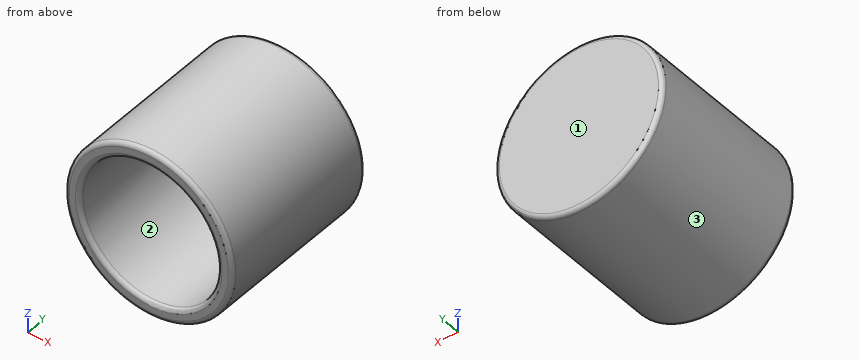
from build123d import *

# Parameters (mm, degrees)
F0_R     = 25.4
F0_R_2   = 20.955
F2_DEPTH = 50.8
F1_R     = 20.955
F3_DEPTH = 12.7
F4_R     = 1.27
F5_R     = 1.27
F6_R     = 1.27


with BuildPart() as f2:
    # F0 (on Front) → F2 (new body)
    with BuildSketch(Plane.XZ):
        Circle(F0_R)
        Circle(F0_R_2, mode=Mode.SUBTRACT)
    extrude(amount=F2_DEPTH)

    # F1 (on face) → F3 (join)
    with BuildSketch(Plane.XZ):
        Circle(F1_R)
    extrude(amount=F3_DEPTH)

    # F4
    f4_edges = [f2.edges().sort_by_distance(p)[0] for p in [
        (-25.4, -50.8, 0),
    ]]
    fillet(f4_edges, radius=F4_R)

    # F5
    f5_edges = [f2.edges().sort_by_distance(p)[0] for p in [
        (-20.955, -50.8, 0),
    ]]
    fillet(f5_edges, radius=F5_R)

    # F6
    f6_edges = [f2.edges().sort_by_distance(p)[0] for p in [
        (-25.4, 0, 0),
    ]]
    fillet(f6_edges, radius=F6_R)


solid = f2.part
Part model, mm, in its own coordinate system. Face numbers are marked on the shaded views. Give positions to 0.01 mm unless a question says otherwise; leave off trailing zeros. Loops run counter-clockwise (first coordinate to the right, second up) from the corner with the lowest first, then second, coordinate; pieces in that order, holes last.
(1) Band-saw the part on B-B (x = 0). Write the cut outline in (y, z) (3 decimals), and give its area (3 significant figures).
Return value:
outline: (-50.8, -24.13) arc R1.27 ccw to (-49.53, -25.4) - (-1.27, -25.4) arc R1.27 ccw to (0, -24.13) - (0, 24.13) arc R1.27 ccw to (-1.27, 25.4) - (-49.53, 25.4) arc R1.27 ccw to (-50.8, 24.13) - (-50.8, 22.225) arc R1.27 ccw to (-49.53, 20.955) - (-12.7, 20.955) - (-12.7, -20.955) - (-49.53, -20.955) arc R1.27 ccw to (-50.8, -22.225) - close
area: 982 mm2
(2) Band-saw the part on A-A (z = 0). Write the cut outline in (x, y) (3 decimals).
Return value:
outline: (-25.4, -49.53) arc R1.27 ccw to (-24.13, -50.8) - (-22.225, -50.8) arc R1.27 ccw to (-20.955, -49.53) - (-20.955, -12.7) - (20.955, -12.7) - (20.955, -49.53) arc R1.27 ccw to (22.225, -50.8) - (24.13, -50.8) arc R1.27 ccw to (25.4, -49.53) - (25.4, -1.27) arc R1.27 ccw to (24.13, 0) - (-24.13, 0) arc R1.27 ccw to (-25.4, -1.27) - close
(3) Band-saw the part on C-C (y = -31). Write the cut outline in (x, z) (3 decimals).
Return value:
outline: circle Ø50.8 at (0, 0); hole circle Ø41.91 at (0, 0)
(4) Drill centre lines: line 1 along Z through (x, y) = (0, -40) (3 decimals); line 2 along Y through (x, z) = (1, 2); line 3 along Y through (x, z) = (17, -14). Where is each one in solid material? Low to high.
Return value:
line 1: z = -25.4 to -20.955, 20.955 to 25.4
line 2: y = -12.7 to 0
line 3: y = -50.78 to 0
(5) Pin check, flat tips, straight feed: pin 1 (1 mm diameter, centred on y = -30.5, z = 18, fed in from +X); pin 2 (3 mm diameter, centred on y = -44, z = 7.5, fed in from -X); pin 3 (3 mm diameter, centred on y = -27.5, z = -7, fed in from -X). Stop position of each tip, or through.
Return value:
pin 1: stops at x = 18.41
pin 2: stops at x = -24.68
pin 3: stops at x = -24.8
(6) Pull direction Z, two halves, no side cores. Call the marked faces 1, 2 and 3: pulls with the +Z half, pulls with the -Z half, needs draft (parallel to the pull), parting line crosses it, or undercut.
Return value:
face 1: needs draft
face 2: undercut
face 3: parting line crosses it
